Read the model definition and answer for the solid it produces. Units are mm, in the model's axes. Give positions to 0.01 mm unless a question says otherwise; leave off trailing zeros. Order: outer loops, then holes, each group sorted by start corner. A loop starts at its lowest first (then second) coordinate and runs counter-clockwise, first axis right, second up.
Item 1: Find the intervals of material crossed by line 1 along Y through (x, z) = (106.5, 2.7); line 2 along X through (y, z) = (59, 0.35); line 3 along X through (y, z) = (102, 2.25), in increasing order.
Item 2: A cutting plane is placed at A-A (y = 90.5). Write down the section's boundary in (x, z), plus the area to 3 significant figures.
Item 3: A cutting plane is placed at B-B (y = 148.5). Write down the section's boundary in (x, z), plus the area to 3 significant figures.
Item 4: A cutting plane is placed at C-C (x = 46). Write down the section's boundary in (y, z).
Item 5: The mould has two halves that part along Y. Classify faces 1 (the face through (90, 8.204, 2)), 2 (the face through (68.314, 128.262, 1.732)), 3 (the face through (91, 158.204, 2)): +Y half, -Y half, draft (parallel to the pull), parting line (faces both ways), or undercut.
Item 6: A cutting plane is placed at D-D (z = 1.25). State how many separate pieces and enclosed holes the cut face has, plus the area to 3 significant figures.
Item 7: Given pin 1 Ø2 at (x, z) = (149, 1.5) entering from +Y, flat-ended and moving along its own axis, determine where the tip first touches the part or whether it passes through.
Autodesk Inventor part; units mm, degrees
ref_plane "YZ Plane" through (0, 0, 0) normal (1, 0, 0) x (0, 1, 0)
ref_plane "XZ Plane" through (0, 0, 0) normal (0, 1, 0) x (-1, 0, 0)
ref_plane "XY Plane" through (0, 0, 0) normal (0, 0, 1) x (1, 0, 0)
sketch "Sketch1" plane through (0, 0, 0) normal (0, 0, 1) x (1, 0, 0)
  line L0 (10.9384, 8.2044) -> (170.9384, 8.2044)
  line L1 (170.9384, 8.2044) -> (170.9384, 98.2044)
  line L2 (10.9384, 98.2044) -> (10.9384, 8.2044)
  line L3 (10.9384, 98.2044) -> (60.9384, 158.2044)
  line L4 (60.9384, 158.2044) -> (120.9384, 158.2044)
  line L5 (120.9384, 158.2044) -> (170.9384, 98.2044)
  dimension "d0" = 160
  dimension "d4" = 60
  dimension "d5" = 50
  dimension "d6" = 90
  dimension "d7" = 90
  dimension "d8" = 150
extrude "Extrusion1" add sketch "Sketch1" along normal blind 3.4163
sketch "Sketch2" plane through (0, 0, 3.4163) normal (0, 0, 1) x (1, 0, 0)
  line L0 (10.9384, 8.2044) -> (10.9384, 98.2044)
  line L1 (170.9384, 8.2044) -> (10.9384, 8.2044)
  circle A0 centre (20.9384, 20.9044) radius 3.57
  circle A1 centre (20.9384, 85.5044) radius 2.625
  dimension "d11" = 7.14
  dimension "d12" = 12.7
  dimension "d13" = 10
  dimension "d14" = 10
  dimension "d15" = 64.6
  dimension "d16" = 5.25
extrude "wheel_holes" cut sketch "Sketch2" against normal through all
pattern_linear "Rectangular Pattern1" count 2 spacing 140 along (1, 0, 0) of "wheel_holes"
sketch "Sketch3" plane through (0, 0, 3.4163) normal (0, 0, 1) x (1, 0, 0)
  line L0 (10.9384, 8.2044) -> (10.9384, 98.2044)
  line L1 (170.9384, 8.2044) -> (10.9384, 8.2044)
  arc A0 (79.4384, 85.5044) -> (102.4384, 85.5044) centre (90.9384, 85.5044) ccw
  arc A1 (73.8194, 100.9984) -> (77.0694, 100.9984) centre (75.4444, 100.9984) ccw
  line L2 (170.9384, 98.2044) -> (170.9384, 8.2044)
  arc A2 (77.0694, 110.9984) -> (73.8194, 110.9984) centre (75.4444, 110.9984) ccw
  line L3 (77.0694, 110.9984) -> (77.0694, 100.9984)
  line L4 (73.8194, 110.9984) -> (73.8194, 100.9984)
  arc A3 (102.4384, 95.5044) -> (79.4384, 95.5044) centre (90.9384, 95.5044) ccw
  line L5 (79.4384, 95.5044) -> (79.4384, 85.5044)
  line L6 (102.4384, 85.5044) -> (102.4384, 95.5044)
  arc A4 (104.8074, 100.9984) -> (108.0574, 100.9984) centre (106.4324, 100.9984) ccw
  arc A5 (108.0574, 110.9984) -> (104.8074, 110.9984) centre (106.4324, 110.9984) ccw
  line L7 (108.0574, 110.9984) -> (108.0574, 100.9984)
  line L8 (104.8074, 110.9984) -> (104.8074, 100.9984)
  arc A6 (73.8194, 70.0104) -> (77.0694, 70.0104) centre (75.4444, 70.0104) ccw
  arc A7 (77.0694, 80.0104) -> (73.8194, 80.0104) centre (75.4444, 80.0104) ccw
  line L9 (77.0694, 80.0104) -> (77.0694, 70.0104)
  line L10 (73.8194, 80.0104) -> (73.8194, 70.0104)
  arc A8 (104.8074, 70.0104) -> (108.0574, 70.0104) centre (106.4324, 70.0104) ccw
  arc A9 (108.0574, 80.0104) -> (104.8074, 80.0104) centre (106.4324, 80.0104) ccw
  line L11 (108.0574, 80.0104) -> (108.0574, 70.0104)
  line L12 (104.8074, 80.0104) -> (104.8074, 70.0104)
  dimension "d22" = 23
  dimension "d23" = 80
  dimension "d24" = 77.3
  dimension "d33" = 3.25
  dimension "d35" = 64.506
  dimension "d36" = 92.794
  dimension "d105" = 10
  dimension "d106" = 64.506
  dimension "d110" = 3.25
  dimension "d112" = 23
  dimension "d113" = 80
  dimension "d114" = 10
  dimension "d126" = 30.988
  dimension "d129" = 30.988
  dimension "d141" = 10
extrude "Nema_17" cut sketch "Sketch3" against normal through all
sketch "Sketch4" plane through (0, 0, 3.4163) normal (0, 0, 1) x (1, 0, 0)
  circle A0 centre (160.9384, 85.5044) radius 2.625
  circle A1 centre (20.9384, 85.5044) radius 2.625
  line L0 (10.9384, 8.2044) -> (10.9384, 98.2044)
  line L1 (170.9384, 98.2044) -> (170.9384, 8.2044)
  circle A2 centre (60.9384, 84.0044) radius 2.625
  circle A3 centre (120.9384, 84.0044) radius 2.625
  dimension "d39" = 50
  dimension "d41" = 5.25
  dimension "d42" = 50
  dimension "d43" = 1.5
  dimension "d44" = 5.25
  dimension "d99" = 1.5
extrude "Idler_Holes" cut sketch "Sketch4" against normal through all contours A2 | A3
sketch "Sketch5" plane through (0, 0, 3.4163) normal (0, 0, 1) x (1, 0, 0)
  line L0 (60.9384, 158.2044) -> (120.9384, 158.2044)
  circle A0 centre (110.9384, 148.2044) radius 2.625
  circle A1 centre (110.9384, 128.2044) radius 2.625
  circle A2 centre (70.9384, 148.2044) radius 2.625
  circle A3 centre (70.9384, 128.2044) radius 2.625
  line L1 (70.9384, 150.8294) -> (110.9384, 150.8294)
  line L2 (110.9384, 145.5794) -> (70.9384, 145.5794)
  line L3 (70.9384, 130.8294) -> (110.9384, 130.8294)
  line L4 (110.9384, 125.5794) -> (70.9384, 125.5794)
  dimension "d47" = 10
  dimension "d48" = 10
  dimension "d49" = 20
  dimension "d50" = 10
  dimension "d51" = 5.25
  dimension "d52" = 5.25
  dimension "d87" = 40
  dimension "d145" = 40
  dimension "d146" = 40
extrude "x-slot" cut sketch "Sketch5" against normal through all
fillet "Fillet2" radius 3.175 6 edges at (120.9384, 158.2044, 1.7082) (60.9384, 158.2044, 1.7082) (170.9384, 98.2044, 1.7082) (170.9384, 8.2044, 1.7082) (10.9384, 98.2044, 1.7082) (10.9384, 8.2044, 1.7082)
sketch "Sketch7" plane through (0, 0, 0) normal (0, 0, -1) x (-1, 0, 0)
  line L0 (-10.9384, 97.0549) -> (-10.9384, 11.3794)
  line L1 (-170.9384, 11.3794) -> (-170.9384, 97.0549)
  line L2 (-14.1134, 8.2044) -> (-167.7634, 8.2044)
  circle A0 centre (-140.9384, 20.9044) radius 2.625
  circle A1 centre (-40.9384, 20.9044) radius 2.625
  dimension "d68" = 5.25
  dimension "d69" = 12.7
  dimension "d70" = 30
  dimension "d71" = 5.25
  dimension "d72" = 30
  dimension "d73" = 12.7
extrude "two_plater" cut sketch "Sketch7" against normal through all
pattern_linear "Rectangular Pattern3" count 2 spacing 61.5 along (0, 1, 0) of "two_plater"
sketch "Sketch8" plane through (0, 0, 3.4163) normal (0, 0, 1) x (1, 0, 0)
  line L0 (167.7634, 8.2044) -> (14.1134, 8.2044)
  line L1 (10.9384, 11.3794) -> (10.9384, 97.0549)
  arc A0 (14.3759, 50.7044) -> (17.5009, 50.7044) centre (15.9384, 50.7044) ccw
  arc A1 (17.5009, 62.7044) -> (14.3759, 62.7044) centre (15.9384, 62.7044) ccw
  line L2 (14.3759, 50.7044) -> (14.3759, 62.7044)
  line L3 (17.5009, 62.7044) -> (17.5009, 50.7044)
  arc A2 (164.3759, 50.7044) -> (167.5009, 50.7044) centre (165.9384, 50.7044) ccw
  arc A3 (167.5009, 62.7044) -> (164.3759, 62.7044) centre (165.9384, 62.7044) ccw
  line L4 (164.3759, 50.7044) -> (164.3759, 62.7044)
  line L5 (167.5009, 62.7044) -> (167.5009, 50.7044)
  point P0 (0, 0)
  dimension "d76" = 3.125
  dimension "d77" = 3.125
  dimension "d78" = 12
  dimension "d79" = 5
  dimension "d80" = 42.5
  dimension "d81" = 3.125
  dimension "d82" = 5
  dimension "d94" = 150
extrude "limit_switches" cut sketch "Sketch8" against normal through all
sketch "Sketch10" plane through (0, 0, 3.4163) normal (0, 0, 1) x (1, 0, 0)
  line L0 (167.7634, 8.2044) -> (14.1134, 8.2044)
  line L1 (170.9384, 97.0549) -> (170.9384, 11.3794)
  arc A0 (70.9384, 20.8294) -> (70.9384, 15.5794) centre (70.9384, 18.2044) ccw
  arc A1 (110.9384, 15.5794) -> (110.9384, 20.8294) centre (110.9384, 18.2044) ccw
  line L2 (70.9384, 20.8294) -> (110.9384, 20.8294)
  line L3 (110.9384, 15.5794) -> (70.9384, 15.5794)
  point P0 (0, 0)
  dimension "d132" = 5.25
  dimension "d133" = 5.25
  dimension "d134" = 10
  dimension "d135" = 10
  dimension "d136" = 40
  dimension "d137" = 40
  dimension "d138" = 60
extrude "Extrusion10" cut sketch "Sketch10" against normal through all
sketch "Sketch11" plane through (0, 0, 3.4163) normal (0, 0, 1) x (1, 0, 0)
  line L0 (62.4255, 158.2044) -> (119.4513, 158.2044)
  line L1 (10.9384, 11.3794) -> (10.9384, 97.0549)
  circle A0 centre (60.9384, 138.2044) radius 2.625
  circle A1 centre (120.9384, 138.2044) radius 2.625
  point P0 (0, 0)
  dimension "d147" = 5.25
  dimension "d148" = 5.25
  dimension "d149" = 60
  dimension "d150" = 20
  dimension "d151" = 20
  dimension "d152" = 50
extrude "Extrusion11" cut sketch "Sketch11" against normal through all
sketch "Sketch13" plane through (0, 0, 3.4163) normal (0, 0, 1) x (1, 0, 0)
  line L0 (10.9384, 11.3794) -> (10.9384, 97.0549)
  arc A0 (102.4384, 95.5044) -> (79.4384, 95.5044) centre (90.9384, 95.5044) ccw
  arc A1 (69.9934, 118.603) -> (64.7015, 119.052) centre (67.3684, 119.0744) ccw
  arc A2 (64.7435, 114.0524) -> (69.9934, 114.0744) centre (67.3684, 114.0744) ccw
  line L1 (69.9934, 118.603) -> (69.9934, 114.0744)
  line L2 (64.7435, 114.0524) -> (64.7015, 119.052)
  point P0 (0, 0)
  dimension "d155" = 5.334
  dimension "d156" = 56.43
  dimension "d157" = 23.57
  dimension "d166" = 5.25
  dimension "d167" = 5
  dimension "d168" = 56.43
extrude "Extrusion12" cut sketch "Sketch13" against normal through all
pattern_linear "Rectangular Pattern4" count 2 spacing 47.14 along (1, 0, 0) count 2 spacing 47.14 along (0, -1, 0) of "Extrusion12"
equation "\"d7\" = d6"
equation "\"d35\" = d29"
equation "\"d112\" = d22"
equation "\"d113\" = d23"
equation "\"d42\" = d39"
equation "\"d43\" = d99"
equation "\"d44\" = d41"
equation "\"d50\" = d48"
equation "\"d52\" = d51"
equation "\"d76\" = d77"
equation "\"d82\" = d79"
equation "\"d134\" = d135"
properties part number "S2_mm" material "Steel, Mild"
Response values:
1. line 1: y = 8.2 to 15.58, 20.83 to 68.39, 81.63 to 99.37, 112.62 to 125.58, 130.83 to 145.58, 150.83 to 158.2
1. line 2: x = 10.94 to 14.38, 17.5 to 164.38, 167.5 to 170.94
1. line 3: x = 14.1 to 73.82, 77.07 to 81.45, 100.43 to 104.81, 108.06 to 167.78
2. outline: (10.94, 0) - (79.44, 0) - (79.44, 3.42) - (10.94, 3.42) - close; (102.44, 0) - (170.94, 0) - (170.94, 3.42) - (102.44, 3.42) - close
2. area: 468 mm2
3. outline: (52.85, 0) - (68.33, 0) - (68.33, 3.42) - (52.85, 3.42) - close; (113.55, 0) - (129.03, 0) - (129.03, 3.42) - (113.55, 3.42) - close
3. area: 106 mm2
4. outline: (8.2, 0) - (140.28, 0) - (140.28, 3.42) - (8.2, 3.42) - close
5. face 1: -Y half
5. face 2: undercut
5. face 3: +Y half
6. separate pieces: 1
6. enclosed holes: 26
6. area: 18,900 mm2
7. pin 1: stops at y = 125.73
